Could you check a few things on this model? Use its own coordinates, in mm. Face numbers are marked on the shaded views. A direction names the side the tool comes from. Coordinates: 2 decimals unless noted, no trailing zeros. Loops run counter-clockwise (first coordinate to the right, second up) from the corner with the lowest first, then second, coordinate; pieces in that order, holes last. Notation, with made-up numbers: M -20.5,-7.75 L 3.5,-7.75 A18 ccw 3.5,13.25 Z; hole C 82,12.25 d5. An arc over 180 degrees is marked long. Use one line per item in the form item = value. Start each with the question number.
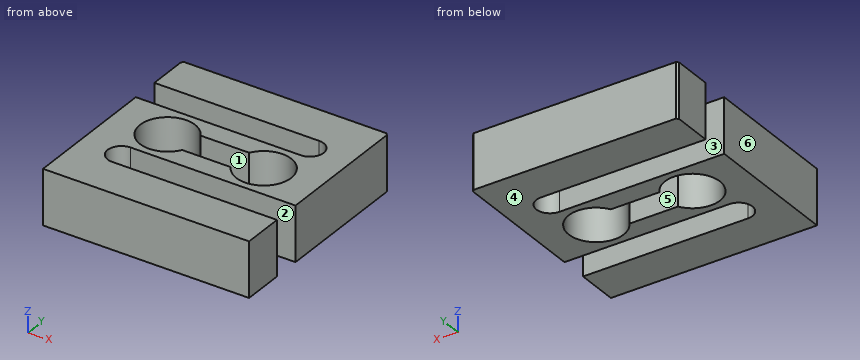
```python
from build123d import *

# Parameters (mm, degrees)
BOSS_EXTRU_1_DEPTH      = 20
ENL_V_MAT_EXTRU_3_DEPTH = 108.935165725


with BuildPart() as part:
    # Esquisse1 → Boss.-Extru.1 (new body)
    with BuildSketch(Plane.XY):
        with BuildLine():
            Line((0, 50), (0, 0))
            Line((0, 0), (75, 0))
            Line((75, 0), (75, 15))
            Line((75, 15), (15, 15))
            ThreePointArc((15, 15), (10, 20), (15, 25))
            Line((15, 25), (75, 25))
            Line((75, 25), (75, 74.292893219))
            Line((75, 74.292893219), (74.292893219, 75))
            Line((74.292893219, 75), (0.707106781, 75))
            Line((0.707106781, 75), (0, 74.292893219))
            Line((0, 74.292893219), (0, 60))
            Line((0, 60), (60, 60))
            ThreePointArc((60, 60), (65, 55), (60, 50))
            Line((60, 50), (0, 50))
        make_face()
    extrude(amount=BOSS_EXTRU_1_DEPTH)

    # Esquisse2 → Enlèv. mat.-Extru.3 (cut, through all)
    with BuildSketch(Plane.XY):
        with BuildLine():
            Line((28.660254038, 42.5), (46.339745962, 42.5))
            ThreePointArc((46.339745962, 42.5), (65, 37.5), (46.339745962, 32.5))
            Line((46.339745962, 32.5), (28.660254038, 32.5))
            ThreePointArc((28.660254038, 32.5), (10, 37.5), (28.660254038, 42.5))
        make_face()
    extrude(amount=ENL_V_MAT_EXTRU_3_DEPTH, mode=Mode.SUBTRACT)


solid = part.part
```
Item 1: Please list where these lines run through material, in increasing order: line 1 along X through (y, z) = (37.5, 6); line 2 along Y through (x, z) = (54.5, 15.75); line 3 along Y through (x, z) = (62, 4.5).
Item 2: For the marked faces 1, 2 and 3, which set-ups out of +Z, -Z, +X, -X, +Y, -Y let a thin tool reach every point of the face, with its end or its side?
Item 3: I want a section at A-A (x = 20). Write out the boundary of the cut face in (y, z).
Item 4: I'm going to push a flat-ended pin straight in: P1, Ø4, axis at x = 53, y = 22.5, coming from the +Z side (3 decimals). Where does the tip first touch, or does it pass through?
Item 5: I want a section at D-D (y = 44). Write out the boundary of the cut face in (x, z).
Item 6: I want a section at C-C (z = 3). Write out the boundary of the cut face in (x, y).
Item 7: Thinking about a two-plate mould opening in X: for the marked faces 4, 5 and 6, which applies, pulls with the +X half, pulls with the -X half, needs draft (parallel to the pull), parting line crosses it, or undercut?
Item 8: I want a section at B-B (x = 5). Write out the boundary of the cut face in (y, z).
Worked answers:
q1.line_1 = 0 to 10, 65 to 75
q1.line_2 = 0 to 15, 25 to 27.51, 47.49 to 50, 60 to 75
q1.line_3 = 0 to 15, 25 to 30.36, 44.64 to 50.42, 59.58 to 75
q2.face_1 = +Z, -Z
q2.face_2 = +Z, -Z, +X
q2.face_3 = +Z, -Z, -X
q3.outline = M 0,0 L 15,0 L 15,20 L 0,20 Z; M 25,0 L 27.5,0 L 27.5,20 L 25,20 Z; M 47.5,0 L 50,0 L 50,20 L 47.5,20 Z; M 60,0 L 75,0 L 75,20 L 60,20 Z
q4.P1 = through
q5.outline = M 0,0 L 12.4,0 L 12.4,20 L 0,20 Z; M 27.6,0 L 47.4,0 L 47.4,20 L 27.6,20 Z; M 62.6,0 L 75,0 L 75,20 L 62.6,20 Z
q6.outline = M 0,0 L 75,0 L 75,15 L 15,15 A5 cw 15,25 L 75,25 L 75,74.29 L 74.29,75 L 0.71,75 L 0,74.29 L 0,60 L 60,60 A5 cw 60,50 L 0,50 Z; hole M 28.66,32.5 L 46.34,32.5 A10 ccw long 46.34,42.5 L 28.66,42.5 A10 ccw long Z
q7.face_4 = needs draft
q7.face_5 = undercut
q7.face_6 = pulls with the -X half
q8.outline = M 0,0 L 50,0 L 50,20 L 0,20 Z; M 60,0 L 75,0 L 75,20 L 60,20 Z
